```python
from build123d import *

# Parameters (mm, degrees)
F1_DEPTH      = 20
F1_DEPTH_BACK = 20
F3_DEPTH      = 10
F3_DEPTH_BACK = 10
F5_DEPTH      = 25
F5_DEPTH_BACK = 25
F6_T4_ANGLE   = 76.4346442218
F6_T10_ANGLE  = 76.4346442218
F6_T16_ANGLE  = 76.4346442218
F6_T22_ANGLE  = 76.4346442218


# Not quite as in the source:
# - a fillet or chamfer that OpenCascade refuses, or shapes differently, is made with other operations: its cross-section is extruded or revolved along the edge and cut away or added
# - two fillets or chamfers of one size are made in one step


with BuildPart() as f1:
    # F0 (on Top) → F1 (new body, two sides)
    with BuildSketch(Plane.XY) as f1_sk:
        with BuildLine():
            Line((11, 0), (24, 0))
            ThreePointArc((24, 0), (0, 24), (-24, 0))
            Line((-24, 0), (-11, 0))
            ThreePointArc((-11, 0), (0, 11), (11, 0))
        make_face()
        with BuildLine():
            ThreePointArc((-24, 0), (0, -24), (24, 0))
            Line((24, 0), (11, 0))
            ThreePointArc((11, 0), (0, -11), (-11, 0))
            Line((-11, 0), (-24, 0))
        make_face()
    extrude(amount=F1_DEPTH)
    extrude(f1_sk.sketch, amount=-F1_DEPTH_BACK)

    # F2 (on Top) → F3 (join, two sides)
    with BuildSketch(Plane.XY) as f3_sk:
        Polygon((-124.000001856, 8), (-124.000001856, 0), (-124.000001856, -8), (-22.981626913, -8), (-22.981626913, 8), align=None)
    extrude(amount=F3_DEPTH)
    extrude(f3_sk.sketch, amount=-F3_DEPTH_BACK)

    # F4 (on Front) → F5 (cut, two sides)
    with BuildSketch(Plane.XZ) as f5_sk:
        with BuildLine():
            Line((-13.159872964, -8.3219918372), (24.1259910374, -8.1159918464))
            Line((24.1259910374, -8.1159918464), (24.037594278, 7.8837639647))
            Line((24.037594278, 7.8837639647), (-13.159872964, 7.8837639647))
            ThreePointArc((-13.159872964, 7.8837639647), (-17.9421277203, -0.2191139363), (-13.159872964, -8.3219918372))
        make_face()
    extrude(amount=-F5_DEPTH, mode=Mode.SUBTRACT)
    extrude(f5_sk.sketch, amount=F5_DEPTH_BACK, mode=Mode.SUBTRACT)

    # F6: fillet of radius 10 on 4 edges, made by hand


with BuildPart() as f6_tool2:
    # F6_s3 → F6_t4 (revolve)
    with BuildSketch(Plane(origin=(0, 0, 0), x_dir=(0, 0, 1), z_dir=(0.9721030029, -0.2345543684, 0))):
        with BuildLine():
            ThreePointArc((20, 24), (12.9289321881, 26.9289321881), (10, 34))
            Line((10, 34), (10, 24))
            Line((10, 24), (20, 24))
        make_face()
    revolve(axis=Axis((0, 0, 10), (0, 0, -1)), revolution_arc=F6_T4_ANGLE)

    split(bisect_by=Plane.XZ.offset(8), keep=Keep.BOTTOM)

    split(bisect_by=Plane.YZ.offset(-22.981626913), keep=Keep.BOTTOM)


with BuildPart() as f1_1:
    add(f1.part)

    # F6_t1: union F6_tool2
    add(f6_tool2.part)


with BuildPart() as f6_tool8:
    # F6_s9 → F6_t10 (revolve)
    with BuildSketch(Plane.XZ):
        with BuildLine():
            ThreePointArc((-24, 20), (-26.9289321881, 12.9289321881), (-34, 10))
            Line((-34, 10), (-24, 10))
            Line((-24, 10), (-24, 20))
        make_face()
    revolve(axis=Axis((0, 0, 10), (0, 0, -1)), revolution_arc=F6_T10_ANGLE)

    split(bisect_by=Plane.XZ.offset(-8), keep=Keep.TOP)

    split(bisect_by=Plane.YZ.offset(-22.981626913), keep=Keep.BOTTOM)


with BuildPart() as f1_2:
    add(f1_1.part)

    # F6_t7: union F6_tool8
    add(f6_tool8.part)


with BuildPart() as f6_tool14:
    # F6_s15 → F6_t16 (revolve)
    with BuildSketch(Plane(origin=(0, 0, 0), x_dir=(0, 0, 1), z_dir=(0.9721030029, 0.2345543684, 0))):
        with BuildLine():
            ThreePointArc((-20, -24), (-12.9289321881, -26.9289321881), (-10, -34))
            Line((-10, -34), (-10, -24))
            Line((-10, -24), (-20, -24))
        make_face()
    revolve(axis=Axis((0, 0, -10), (0, 0, 1)), revolution_arc=F6_T16_ANGLE)

    split(bisect_by=Plane.XZ.offset(-8), keep=Keep.TOP)

    split(bisect_by=Plane.YZ.offset(-22.981626913), keep=Keep.BOTTOM)


with BuildPart() as f1_3:
    add(f1_2.part)

    # F6_t13: union F6_tool14
    add(f6_tool14.part)


with BuildPart() as f6_tool20:
    # F6_s21 → F6_t22 (revolve)
    with BuildSketch(Plane.XZ):
        with BuildLine():
            ThreePointArc((-24, -20), (-26.9289321881, -12.9289321881), (-34, -10))
            Line((-34, -10), (-24, -10))
            Line((-24, -10), (-24, -20))
        make_face()
    revolve(axis=Axis((0, 0, -10), (0, 0, 1)), revolution_arc=F6_T22_ANGLE)

    split(bisect_by=Plane.XZ.offset(8), keep=Keep.BOTTOM)

    split(bisect_by=Plane.YZ.offset(-22.981626913), keep=Keep.BOTTOM)


with BuildPart() as f1_4:
    add(f1_3.part)

    # F6_t19: union F6_tool20
    add(f6_tool20.part)


solid = f1_4.part
```
The listing builds one solid part. Answer for the finished solid, in the listing's coordinates (mm). A direction names the side the tool comes from. Coordinates: 2 decimals unless noted, no trailing zeros. Order: outer loops, then holes, each group sorted by start corner. A loop starts at its lowest first (then second) coordinate and runs counter-clockwise, first axis right, second up. Notation, with made-up numbers: M 38.5,42 L 51.5,42 A25 ccw 51.5,59 Z; hole C 65,-12.5 d1. An arc over 180 degrees is marked long. Answer as a JSON object with one key per item and string values. Group by question number.
1. Section A-A on x = 14 is taken. Write down the section's boundary in (y, z).
2. Section C-C on z = -11.5 is taken. Write down the section's boundary in (x, y), then the cut area to 3 significant figures.
3. Determine the mould class of faces 1 (the cylindrical face through (-2.38, 10.74, 14.03)), 2 (the flat face through (-74, -8, 0)), 3 (the flat face through (-124, 0, 0)), 4 (the cylindrical face through (-2.38, 10.74, -14.01)) for opening direction X: released by +X, released by -X, zero draft, split by the parting line, or undercut.
4. Flat-ended cylindrical pins translate along their axes: P1, Ø5, axis at x = -89, z = -0.5, coming from the +Y side; P2, Ø10, axis at x = -72, y = 0, coming from the -Z side; P3, Ø12, axis at y = -18.5, z = 6, coming from the -X side; P4, Ø11, axis at x = 4.5, y = 2.5, coming from the -Z side. Find the tip coordinate at first contact, or state that the pin passes through.
5. Straight lines are drawn through the part: line 1 (Y direction, x = 0, z = 10.5); line 2 (Z direction, x = 5.5, y = 14.5); line 3 (Z direction, x = 18.5, y = -1). For each, find the intervals that lie inside material, in ascending order.
6. Section B-B on y = 21.5 is taken. Write down the section's boundary in (x, z).
7. A tool of negligible diameter and unlimited length cuts with its end or side. For faces 5 (the flat face through (-74, 8, 0)), 6 (the flat face through (-79, 0, -10)), 7 (the flat face through (-79, 0, 10)), 8 (the flat face through (10, 5, 7.884)), from which of +Z, -Z, +X, -X, +Y, -Y can it reach the whole face along a straight path? Write none if from no direction.
8. Section D-D on y = -14 is taken. Write down the section's boundary in (x, z).
Values follow:
{
 "1": {"outline": "M -19.49,-20 L 19.49,-20 L 19.49,-8.17 L -19.49,-8.17 Z; M -19.49,7.88 L 19.49,7.88 L 19.49,20 L -19.49,20 Z"},
 "2": {"outline": "M -27.6,-8 L -22.98,-8 L -22.98,-6.92 A24 ccw long -22.98,6.92 L -22.98,8 L -27.6,8 A28.73 ccw Z; hole C 0,0 d22", "area": "1,510 mm2"},
 "3": {"face 1": "undercut", "face 2": "zero draft", "face 3": "released by -X", "face 4": "undercut"},
 "4": {"P1": "y = 8", "P2": "z = -10", "P3": "x = -20.49", "P4": "through"},
 "5": {"line 1": "-24 to -11, 11 to 24", "line 2": "-20 to -8.22, 7.88 to 20", "line 3": "-20 to -8.15, 7.88 to 20"},
 "6": {"outline": "M -10.67,-20 L 10.67,-20 L 10.67,-8.19 L -10.67,-8.31 Z; M -10.67,7.88 L 10.67,7.88 L 10.67,20 L -10.67,20 Z"},
 "7": {"face 5": "+Z, -Z, -X, +Y", "face 6": "-Z, -X, +Y, -Y", "face 7": "+Z, -X, +Y, -Y", "face 8": "+X, +Y, -Y"},
 "8": {"outline": "M -19.49,-20 L 19.49,-20 L 19.49,-8.14 L -13.16,-8.32 A9.26 cw -13.16,7.88 L 19.49,7.88 L 19.49,20 L -19.49,20 Z"}
}
